Model file for the job. Use its own axes, mm. Face numbers are marked on the shaded views. A direction names the side the tool comes from. Coordinates: 2 decimals unless noted, no trailing zeros. Order: outer loops, then holes, each group sorted by start corner. A loop starts at its lowest first (then second) coordinate and runs counter-clockwise, first axis right, second up. Notation, with made-up numbers: (46, -8) -> (87, -8) arc R17 cw to (87, 10) -> close; hole circle Ø11 at (25, 22). An arc over 180 degrees is marked (long way). Return JSON: item names as keys, results as strings. Group by question number.
1) Cut at C-C (x = -73.5). Write the cut outline in (y, z), and give its area (3 significant figures).
2) Probe line 1 (X direction, y = 5, z = -52); line 2 (Y direction, x = -61.5, z = -56); line 3 (Y direction, x = -53.5, z = -65.5). List the from-to ranges inside material, lowest first.
3) Which spindle directions (+Z, -Z, +X, -X, +Y, -Y) get a long thin tool onto all of the face, cutting with end or side? Do the marked faces 4 and 5. Say none if no direction does.
4) Cut at D-D (y = 5.25). Write the cut outline in (x, z).
5) Cut at A-A (y = 16). Write the cut outline in (x, z).
6) Cut at B-B (z = -60.5). Write the cut outline in (x, y).
7) Flat gauge pins, fed straight in: pin 1 (1.6 mm diameter, centred on x = -16, y = 16, fed in from -Z); pin 2 (0.8 mm diameter, centred on y = 16, z = -52, fed in from +X); pin 3 (1.2 mm diameter, centred on x = -13, y = 16, fed in from +Z). Where does each tip first touch, or does it go through?
8) Pull direction Z, two halves, no side cores. Call the marked faces 1, 2 and 3: +Z half, -Z half, draft (parallel to the pull), parting line (faces both ways), or undercut.
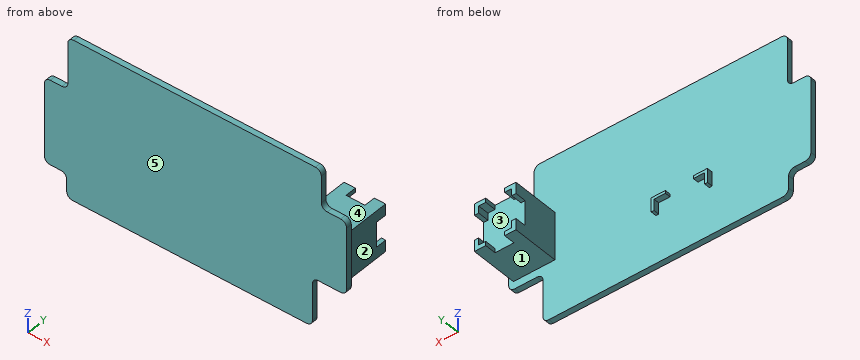
from build123d import *

# Parameters (mm, degrees)
BOSS_EXTRUDE1_DEPTH = 2
BOSS_EXTRUDE2_DEPTH = 2
SKETCH3_W           = 14.7
SKETCH3_H           = 16.85
BOSS_EXTRUDE3_DEPTH = 12.75
BOSS_EXTRUDE4_DEPTH = 4


with BuildPart() as part:
    # Sketch1 → Boss-Extrude1 (new body)
    with BuildSketch(Plane(origin=(0, 0, 0), x_dir=(1, 0, 0), z_dir=(0, 1, 0))):
        with BuildLine():
            Line((-14.340002267, 86.923975611), (-97.140002267, 86.923975611))
            ThreePointArc((-97.140002267, 86.923975611), (-98.624926507, 86.308899852), (-99.240002267, 84.823975611))
            Line((-99.240002267, 84.823975611), (-99.240002267, 80.522464507))
            ThreePointArc((-99.240002267, 80.522464507), (-99.855078026, 79.037540266), (-101.340002267, 78.422464507))
            Line((-101.340002267, 78.422464507), (-105.03337779, 78.422464507))
            ThreePointArc((-105.03337779, 78.422464507), (-106.51830203, 77.807388747), (-107.13337779, 76.322464507))
            Line((-107.13337779, 76.322464507), (-107.13337779, 50.522464507))
            ThreePointArc((-107.13337779, 50.522464507), (-106.51830203, 49.037540266), (-105.03337779, 48.422464507))
            Line((-105.03337779, 48.422464507), (-100.956274126, 48.422464507))
            ThreePointArc((-100.956274126, 48.422464507), (-99.471349885, 47.807388747), (-98.856274126, 46.322464507))
            Line((-98.856274126, 46.322464507), (-98.856274126, 32.023975611))
            ThreePointArc((-98.856274126, 32.023975611), (-98.241198366, 30.539051371), (-96.756274126, 29.923975611))
            Line((-96.756274126, 29.923975611), (-11.195092997, 29.923975611))
            ThreePointArc((-11.195092997, 29.923975611), (-9.710168757, 30.539051371), (-9.095092997, 32.023975611))
            Line((-9.095092997, 32.023975611), (-9.095092997, 41.509498791))
            ThreePointArc((-9.095092997, 41.509498791), (-8.480017238, 42.994423032), (-6.995092997, 43.609498791))
            Line((-6.995092997, 43.609498791), (-2.23337779, 43.609498791))
            ThreePointArc((-2.23337779, 43.609498791), (-0.748453549, 44.224574551), (-0.13337779, 45.709498791))
            Line((-0.13337779, 45.709498791), (-0.13337779, 67.540883484))
            ThreePointArc((-0.13337779, 67.540883484), (-0.748453549, 69.025807724), (-2.23337779, 69.640883484))
            Line((-2.23337779, 69.640883484), (-10.140002267, 69.640883484))
            ThreePointArc((-10.140002267, 69.640883484), (-11.624926507, 70.255959243), (-12.240002267, 71.740883484))
            Line((-12.240002267, 71.740883484), (-12.240002267, 84.823975611))
            ThreePointArc((-12.240002267, 84.823975611), (-12.855078026, 86.308899852), (-14.340002267, 86.923975611))
        make_face()
    extrude(amount=BOSS_EXTRUDE1_DEPTH)

    # Sketch2 → Boss-Extrude2 (add)
    with BuildSketch(Plane(origin=(0, 2, 0), x_dir=(1, 0, 0), z_dir=(0, 1, 0))):
        Polygon((-52.240002267, 64.923975611), (-57.240002267, 64.923975611), (-57.240002267, 65.923975611), (-53.240002267, 65.923975611), (-53.240002267, 69.923975611), (-52.240002267, 69.923975611), align=None)
        Polygon((-72.140002267, 64.923975611), (-67.140002267, 64.923975611), (-67.140002267, 65.923975611), (-71.140002267, 65.923975611), (-71.140002267, 69.923975611), (-72.140002267, 69.923975611), align=None)
    extrude(amount=BOSS_EXTRUDE2_DEPTH)

    # Sketch3 → Boss-Extrude3 (add)
    with BuildSketch(Plane(origin=(0, 2, 0), x_dir=(1, 0, 0), z_dir=(0, 1, 0))):
        with Locations((-9.13337779, 58.423975611)):
            Rectangle(SKETCH3_W, SKETCH3_H)
    extrude(amount=BOSS_EXTRUDE3_DEPTH)

    # Sketch4 → Boss-Extrude4 (add)
    with BuildSketch(Plane(origin=(0, 14.75, 0), x_dir=(1, 0, 0), z_dir=(0, 1, 0))):
        Polygon((-1.78337779, 49.998975611), (-5.78337779, 49.998975611), (-5.78337779, 51.498975611), (-3.28337779, 51.498975611), (-3.28337779, 53.998975611), (-1.78337779, 53.998975611), align=None)
        Polygon((-1.78337779, 66.848975611), (-5.78337779, 66.848975611), (-5.78337779, 65.348975611), (-3.28337779, 65.348975611), (-3.28337779, 62.848975611), (-1.78337779, 62.848975611), align=None)
        Polygon((-16.48337779, 49.998975611), (-16.48337779, 53.998975611), (-14.98337779, 53.998975611), (-14.98337779, 51.498975611), (-12.48337779, 51.498975611), (-12.48337779, 49.998975611), align=None)
        Polygon((-14.98337779, 62.848975611), (-16.48337779, 62.848975611), (-16.48337779, 66.848975611), (-12.48337779, 66.848975611), (-12.48337779, 65.348975611), (-14.98337779, 65.348975611), align=None)
    extrude(amount=BOSS_EXTRUDE4_DEPTH)


solid = part.part
Answers below:
{
 "1": {"outline": "(0, -86.92) -> (2, -86.92) -> (2, -29.92) -> (0, -29.92) -> close", "area": "114 mm^2"},
 "2": {"line 1": "x = -16.48 to -1.78", "line 2": "y = 0 to 2", "line 3": "y = 0 to 4"},
 "3": {"face 4": "+Z, +X, -X, +Y", "face 5": "+Z, -Z, +X, -X, -Y"},
 "4": {"outline": "(-16.48, -66.85) -> (-1.78, -66.85) -> (-1.78, -50) -> (-16.48, -50) -> close"},
 "5": {"outline": "(-16.48, -66.85) -> (-12.48, -66.85) -> (-12.48, -65.35) -> (-14.98, -65.35) -> (-14.98, -62.85) -> (-16.48, -62.85) -> close; (-16.48, -54) -> (-14.98, -54) -> (-14.98, -51.5) -> (-12.48, -51.5) -> (-12.48, -50) -> (-16.48, -50) -> close; (-5.78, -66.85) -> (-1.78, -66.85) -> (-1.78, -62.85) -> (-3.28, -62.85) -> (-3.28, -65.35) -> (-5.78, -65.35) -> close; (-5.78, -51.5) -> (-3.28, -51.5) -> (-3.28, -54) -> (-1.78, -54) -> (-1.78, -50) -> (-5.78, -50) -> close"},
 "6": {"outline": "(-107.13, 0) -> (-0.13, 0) -> (-0.13, 2) -> (-1.78, 2) -> (-1.78, 14.75) -> (-16.48, 14.75) -> (-16.48, 2) -> (-107.13, 2) -> close"},
 "7": {"pin 1": "stops at z = -66.85", "pin 2": "stops at x = -1.78", "pin 3": "stops at z = -50"},
 "8": {"face 1": "-Z half", "face 2": "draft", "face 3": "undercut"}
}
